For this review, take the finished solid that the model builds, in its own axes (mm). A direction names the side the tool comes from. Give positions to 0.01 mm unless a question says otherwise; leave off trailing zeros. Write each loop counter-clockwise with the first axis right and the second up, starting at its lowest first coordinate (ties: lowest second). Pieces come first, ordered by that corner, then holes. Notation, with made-up numbers: M 8.25,74 L 51.25,74 A29 cw 51.25,106 Z; hole C 73,63 d2. An arc over 180 degrees is marked long. One line per item, written item: value. Start each with the question number.
Item 1: Clearance check with flat-ended pins moving along their axes: pin 1 Ø20.5 at (x, z) = (28.5, 89) entering from -Y; pin 2 Ø12.5 at (y, z) = (46, 8) entering from +X; pin 3 Ø8 at (y, z) = (30.5, 51) entering from +X. State where each tip first meets the part, or that it passes through.
Item 2: To check wall thickness, follow probe 1 along Y at (x, z) = (113, 23); probe 2 along X at (y, z) = (39, 24.5); probe 3 along X at (y, z) = (74.5, 45.5). State the ranges of each line that lie inside material, in increasing order.
Item 3: Consider section A-A, the plane x = 114. Write out the cut boundary in (y, z), and give its area (3 significant figures).
Item 4: Mouldability with a two-part tool opening along Y and no side actions: class faces 6 (the face through (145.16, 89.08, 17.76)), 7 (the face through (127, 76.2, 13)), 8 (the face through (58, 101.6, 21)), 9 (the face through (25.76, 7.64, 94.36)) as released by +Y, released by -Y, zero draft, split by the parting line, or undercut.
Item 5: Consider section B-B, the plane z = 95.5. Write out the cut boundary in (x, y).
Item 6: Tool access review of faces 1 (the face through (101.6, 50, 13)), 2 (the face through (0, 50, 39)), 3 (the face through (50.8, 50, 46)), 4 (the face through (58, 52, 0)), 5 (the face through (26, 76.2, 89)): name each direction out of +Z, -Z, +X, -X, +Y, -Y from which nothing blocks a thin tool from reaching the whole face with its end or side.
```python
from build123d import *

# Parameters (mm, degrees)
F0_W     = 152.4
F0_H     = 101.6
F1_DEPTH = 25.4
F2_W     = 50.8
F2_H     = 50.8
F3_DEPTH = 25.401
F4_W     = 50.8
F4_H     = 101.6
F5_DEPTH = 76.2
F6_W     = 50.8
F6_H     = 25.4
F7_DEPTH = 50.801
F9_DEPTH = 50.801
F10_R    = 25.39999


# Not quite as in the source:
# - a fillet or chamfer is up to 0.001 mm smaller than in the source, because OpenCascade refuses the exact size


with BuildPart() as f1:
    # F0 (on Top) → F1 (new body)
    with BuildSketch(Plane.XY):
        with Locations((76.2, 50.8)):
            Rectangle(F0_W, F0_H)
    extrude(amount=F1_DEPTH)

    # F2 (on face) → F3 (cut, through all)
    with BuildSketch(Plane.XY.offset(25.4)):
        with Locations((127, 50.8)):
            Rectangle(F2_W, F2_H)
    extrude(amount=-F3_DEPTH, mode=Mode.SUBTRACT)

    # F4 (on face) → F5 (join)
    with BuildSketch(Plane.XY.offset(25.4)):
        with Locations((25.4, 50.8)):
            Rectangle(F4_W, F4_H)
    extrude(amount=F5_DEPTH)

    # F6 (on face) → F7 (cut, through all)
    with BuildSketch(Plane.YZ.offset(50.8)):
        with Locations((50.8, 88.9)):
            Rectangle(F6_W, F6_H)
    extrude(amount=-F7_DEPTH, mode=Mode.SUBTRACT)

    # F8 (on face) → F9 (cut, through all)
    with BuildSketch(Plane.YZ.offset(50.8)):
        with BuildLine():
            Line((76.2, 76.2), (25.4, 76.2))
            ThreePointArc((25.4, 76.2), (50.8, 50.8), (76.2, 76.2))
        make_face()
    extrude(amount=-F9_DEPTH, mode=Mode.SUBTRACT)

    # F10 (radius 25.4 in the source; OpenCascade refuses exactly that, so slightly less here)
    f10_edges = [f1.edges().sort_by_distance(p)[0] for p in [
        (25.4, 0, 101.6),
        (25.4, 101.6, 101.6),
        (152.4, 12.7, 25.4),
        (152.4, 88.9, 25.4),
    ]]
    fillet(f10_edges, radius=F10_R)


solid = f1.part
```
Model answer:
1. pin 1: stops at y = 0.13
1. pin 2: stops at x = 101.6
1. pin 3: stops at x = 50.8
2. probe 1: y = 0 to 25.4, 76.2 to 101.6
2. probe 2: x = 0 to 101.6
2. probe 3: x = 0 to 50.8
3. outline: M 0,0 L 25.4,0 L 25.4,25.4 L 0,25.4 Z; M 76.2,0 L 101.6,0 L 101.6,25.4 L 76.2,25.4 Z
3. area: 1,290 mm2
4. face 6: zero draft
4. face 7: undercut
4. face 8: released by +Y
4. face 9: released by -Y
5. outline: M 0,8.89 L 50.8,8.89 L 50.8,25.4 L 0,25.4 Z; M 0,76.2 L 50.8,76.2 L 50.8,92.71 L 0,92.71 Z
6. face 1: +Z, -Z, +X
6. face 2: +Z, -Z, -X, +Y, -Y
6. face 3: +Z, +X, +Y, -Y
6. face 4: -Z, +X, -X, +Y, -Y
6. face 5: +Z, +X, -X
